```python
from build123d import *

# Parameters (mm, degrees)
F1_DEPTH = 300
F3_DEPTH = 60
F5_DEPTH = 60


with BuildPart() as f1:
    # F0 (on Top) → F1 (new body)
    with BuildSketch(Plane.XY):
        with BuildLine():
            Line((20, 15), (0, 15))
            Line((0, 15), (-20, 15))
            ThreePointArc((-20, 15), (-35, 0), (-20, -15))
            Line((-20, -15), (0, -15))
            Line((0, -15), (20, -15))
            ThreePointArc((20, -15), (35, 0), (20, 15))
        make_face()
    extrude(amount=F1_DEPTH)

    # F2 (on face) → F3 (cut)
    with BuildSketch(Plane.XY.offset(300)):
        Polygon((-10, 10), (-20, 10), (-20, -18.429138), (0, -18.429138), (20, -18.429138), (20, 10), (10, 10), (10, -5), (0, -5), (-10, -5), align=None)
    extrude(amount=-F3_DEPTH, mode=Mode.SUBTRACT)

    # F4 (on face) → F5 (cut)
    with BuildSketch(Plane(origin=(0, 0, 0), x_dir=(1, 0, 0), z_dir=(0, 0, -1))):
        Polygon((10, -10), (20, -10), (20, 20.498224), (0, 20.498224), (-20, 20.498224), (-20, -10), (-10, -10), (-10, 5), (0, 5), (10, 5), align=None)
    extrude(amount=-F5_DEPTH, mode=Mode.SUBTRACT)


solid = f1.part
```
Can you work these out from the model? Positions are in its coordinate system, mm. A direction names the side the tool comes from. Coordinates: 2 decimals unless noted, no trailing zeros. Order: outer loops, then holes, each group sorted by start corner. A loop starts at its lowest first (then second) coordinate and runs counter-clockwise, first axis right, second up. Notation, with made-up numbers: (5, 77.25) - (35, 77.25) arc R13 ccw to (35, 85.25) - close; hole circle Ø3 at (21.25, 73.25). An arc over 180 degrees is marked (long way). Answer in a Markdown table with one row per item.
1. Suppose I cut it at D-D (z = 109). Please give me the cut outline in (x, y).
Reply:
| item | result |
|---|---|
| outline | (-20, -15) - (20, -15) arc R15 ccw to (20, 15) - (-20, 15) arc R15 ccw to start |
2. For faces 5 (the flat face through (0, 4, 0)), 6 (the flat face through (20, -2, 30)), 7 (the flat face through (-20, -2, 270)), which set-ups out of +Z, -Z, +X, -X, +Y, -Y let a thin tool reach every point of the face, with its end or its side?
Reply:
| item | result |
|---|---|
| face 5 | -Z, +X, -X, +Y, -Y |
| face 6 | -Z, -Y |
| face 7 | +Z, -Y |
3. If I drill on line 1 along X through (y, z) = (1, 277); line 2 along X through (y, z) = (8, 282.5); line 3 along Y through (x, z) = (-8.5, 12), over which ranges is the centre line in solid material (lowest first)?
Reply:
| item | result |
|---|---|
| line 1 | x = -34.97 to -20, -10 to 10, 20 to 34.97 |
| line 2 | x = -32.69 to -20, -10 to 10, 20 to 32.69 |
| line 3 | y = -5 to 15 |
4. Suppose I cut it at B-B (z = 26). Please give me the cut outline in (x, y).
Reply:
| item | result |
|---|---|
| outline | (-20, -15) - (-20, 10) - (-10, 10) - (-10, -5) - (10, -5) - (10, 10) - (20, 10) - (20, -15) arc R15 ccw to (20, 15) - (-20, 15) arc R15 ccw to start |
5. For pin 1 (12.5 mm diameter, centred on x = 9.5, y = -8.5, fed in from +Z); pin 2 (3 mm diameter, centred on x = -14.5, z = 255, fed in from -Y); pin 3 (10 mm diameter, centred on x = -2, z = 41, fed in from -Y); pin 4 (5 mm diameter, centred on y = 9, z = 163, fed in from -X), each with a flat end and sliding along its axis, tell me the tip position at first contact or that it passes through.
Reply:
| item | result |
|---|---|
| pin 1 | stops at z = 300 |
| pin 2 | stops at y = 10 |
| pin 3 | stops at y = -5 |
| pin 4 | stops at x = -33.52 |
6. Suppose I cut it at A-A (x = -5.5). Please give me the cut outline in (y, z), and give its area (3 significant figures).
Reply:
| item | result |
|---|---|
| outline | (-15, 60) - (-5, 60) - (-5, 0) - (15, 0) - (15, 300) - (-5, 300) - (-5, 240) - (-15, 240) - close |
| area | 7,800 mm^2 |
7. If we mould it in two halves opening along X, with no side actions, what happens to faces 1 (the cylindrical face through (35, 0, 148)), 2 (the flat face through (0, 15, 148)), 3 (the cylindrical face through (-35, 0, 148)), 4 (the flat face through (15, 10, 30))? For each: pulls with the +X half, pulls with the -X half, needs draft (parallel to the pull), parting line crosses it, or undercut.
Reply:
| item | result |
|---|---|
| face 1 | pulls with the +X half |
| face 2 | needs draft |
| face 3 | pulls with the -X half |
| face 4 | undercut |
8. Suppose I cut it at C-C (y = -0.5). Please give me the cut outline in (x, z), and give its area (3 significant figures).
Reply:
| item | result |
|---|---|
| outline | (-34.99, 0) - (-20, 0) - (-20, 60) - (-10, 60) - (-10, 0) - (10, 0) - (10, 60) - (20, 60) - (20, 0) - (34.99, 0) - (34.99, 300) - (20, 300) - (20, 240) - (10, 240) - (10, 300) - (-10, 300) - (-10, 240) - (-20, 240) - (-20, 300) - (-34.99, 300) - close |
| area | 18,600 mm^2 |
